Verification items for this drawing (mm, ordinates from the low corner). A direction names the side the tool comes from. Coordinates: 2 decimals unless noted, no trailing zeros. Write each loop counter-clockwise with the first axis right and the second up, starting at its lowest first coordinate (ties: lowest second). Pieces come first, ordered by that corner, then holes. Notation, with made-up numbers: (-24.75, 3.5) -> (-14.75, 3.5) arc R23 ccw to (-14.75, 34.5) -> close; hole circle Ø5 at (70, -18). An arc over 180 degrees is marked (long way). One line per question, with ' | ' between items.
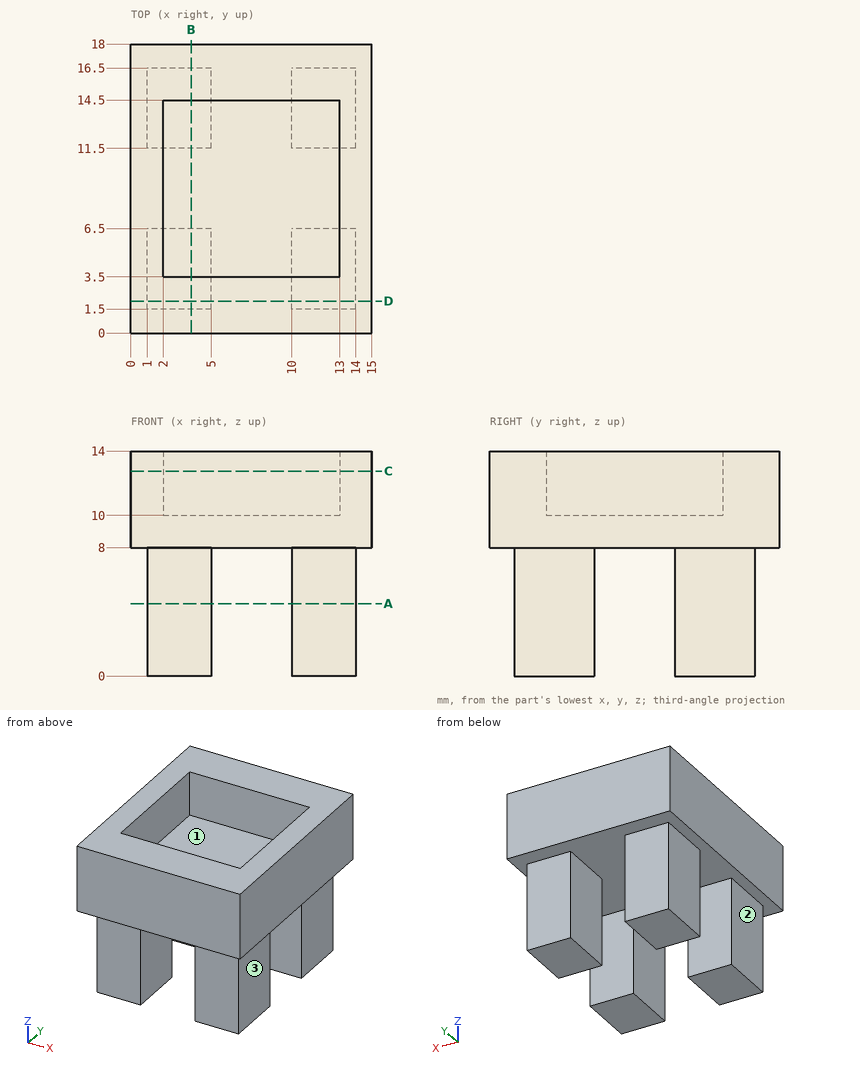
(1) Cross-section at C-C (z = 12.75). Record the cut outline in (x, y), plus the area to 3 significant figures.
Answers below:
outline: (0, 0) -> (15, 0) -> (15, 18) -> (0, 18) -> close; hole (2, 3.5) -> (13, 3.5) -> (13, 14.5) -> (2, 14.5) -> close | area: 149 mm²
(2) Cross-section at D-D (y = 2). Record the cut outline in (x, z), plus the area to 3 significant figures.
Answers below:
outline: (0, 8) -> (1, 8) -> (1, 0) -> (5, 0) -> (5, 8) -> (10, 8) -> (10, 0) -> (14, 0) -> (14, 8) -> (15, 8) -> (15, 14) -> (0, 14) -> close | area: 154 mm²
(3) Depth check by flat-ended pin: P1, Ø2, axis at x = 13, z = 2.5, coming from the -Y side; P2, Ø8, axis at y = 13, z = 4.5, coming from the +X side; P3, Ø4, axis at y = 3.5, z = 3, coming from the +X side; P4, Ø4.5, axis at x = 4, z = 4, coming from the +Y side. Enter the tip coordinate at first touch or a pass-through.
Answers below:
P1: stops at y = 1.5 | P2: stops at x = 15 | P3: stops at x = 14 | P4: stops at y = 16.5
(4) Cross-section at B-B (x = 3.75). Record the cut outline in (y, z), plus the area to 3 significant figures.
Answers below:
outline: (0, 8) -> (1.5, 8) -> (1.5, 0) -> (6.5, 0) -> (6.5, 8) -> (11.5, 8) -> (11.5, 0) -> (16.5, 0) -> (16.5, 8) -> (18, 8) -> (18, 14) -> (14.5, 14) -> (14.5, 10) -> (3.5, 10) -> (3.5, 14) -> (0, 14) -> close | area: 144 mm²
(5) Tool access check on the marked faces 1, 2 and 3. Record the directions out of +Z, -Z, +X, -X, +Y, -Y that give a thin tool (end or side, any length) a straight path to the whole face; none if there is none.
Answers below:
face 1: +Z | face 2: -Z, -X, +Y, -Y | face 3: -Z, +X, +Y, -Y
(6) Cross-section at A-A (z = 4.5). Record the cut outline in (x, y), plus the area to 3 significant figures.
Answers below:
outline: (1, 1.5) -> (5, 1.5) -> (5, 6.5) -> (1, 6.5) -> close; (1, 11.5) -> (5, 11.5) -> (5, 16.5) -> (1, 16.5) -> close; (10, 1.5) -> (14, 1.5) -> (14, 6.5) -> (10, 6.5) -> close; (10, 11.5) -> (14, 11.5) -> (14, 16.5) -> (10, 16.5) -> close | area: 80.0 mm²
(7) Material ranges on line 1 (X direction, y = 15.25, z = 6.75); line 2 (Y direction, x = 13.5, z = 2.25); line 3 (Y direction, x = 6.5, z = 10.5), recorded low to high.
Answers below:
line 1: x = 1 to 5, 10 to 14 | line 2: y = 1.5 to 6.5, 11.5 to 16.5 | line 3: y = 0 to 3.5, 14.5 to 18
